from build123d import *

# Parameters (mm, degrees)
CROQUIS1_W              = 109.11
CROQUIS1_H              = 92
SALIENTE_EXTRUIR1_DEPTH = 32
CROQUIS2_W              = 86
CROQUIS2_H              = 27
CORTAR_EXTRUIR1_DEPTH   = 123.658029089
CORTAR_EXTRUIR2_DEPTH   = 107.753210842
CORTAR_EXTRUIR4_DEPTH   = 77.297103648


with BuildPart() as part:
    # Croquis1 → Saliente-Extruir1 (new body)
    with BuildSketch(Plane(origin=(0, 0, 0), x_dir=(1, 0, 0), z_dir=(0, 1, 0))):
        Rectangle(CROQUIS1_W, CROQUIS1_H)
    extrude(amount=SALIENTE_EXTRUIR1_DEPTH)

    # Croquis2 → Cortar-Extruir1 (cut, through all)
    with BuildSketch(Plane(origin=(54.555, 0, 0), x_dir=(0, 0, -1), z_dir=(1, 0, 0))):
        with Locations((-3, 18.5)):
            Rectangle(CROQUIS2_W, CROQUIS2_H)
    extrude(amount=-CORTAR_EXTRUIR1_DEPTH, mode=Mode.SUBTRACT)

    # Croquis3 → Cortar-Extruir2 (cut, through all)
    with BuildSketch(Plane.XY.offset(-40)):
        with BuildLine():
            Line((45.735, 28.9), (54.555, 28.9))
            Line((54.555, 28.9), (54.555, 25.1))
            Line((54.555, 25.1), (45.735, 25.1))
            ThreePointArc((45.735, 25.1), (43.835, 27), (45.735, 28.9))
        make_face()
        with BuildLine():
            Line((-45.735, 28.9), (-54.555, 28.9))
            Line((-54.555, 28.9), (-54.555, 25.1))
            Line((-54.555, 25.1), (-45.735, 25.1))
            ThreePointArc((-45.735, 25.1), (-43.835, 27), (-45.735, 28.9))
        make_face()
    extrude(amount=-CORTAR_EXTRUIR2_DEPTH, mode=Mode.SUBTRACT)

    # Croquis4 → Cortar-Extruir4 (cut, through all)
    with BuildSketch(Plane(origin=(0, 5, 0), x_dir=(1, 0, 0), z_dir=(0, 1, 0))):
        with BuildLine():
            Line((-46.015, 36), (-54.555, 36))
            Line((-54.555, 36), (-54.555, 31.26))
            Line((-54.555, 31.26), (-46.015, 31.26))
            ThreePointArc((-46.015, 31.26), (-43.645, 33.63), (-46.015, 36))
        make_face()
        with BuildLine():
            Line((-46.015, 17), (-54.555, 17))
            Line((-54.555, 17), (-54.555, 12.26))
            Line((-54.555, 12.26), (-46.015, 12.26))
            ThreePointArc((-46.015, 12.26), (-43.645, 14.63), (-46.015, 17))
        make_face()
        with BuildLine():
            Line((-46.015, -33.037861791), (-54.555, -33.037861791))
            Line((-54.555, -33.037861791), (-54.555, -37.615607647))
            Line((-54.555, -37.615607647), (-46.015, -37.615607647))
            ThreePointArc((-46.015, -37.615607647), (-43.726127072, -35.326734719), (-46.015, -33.037861791))
        make_face()
        with BuildLine():
            Line((54.555, -37.615607647), (46.015, -37.615607647))
            ThreePointArc((46.015, -37.615607647), (43.726127072, -35.326734719), (46.015, -33.037861791))
            Line((46.015, -33.037861791), (54.555, -33.037861791))
            Line((54.555, -33.037861791), (54.555, -37.615607647))
        make_face()
        with BuildLine():
            Line((54.555, 17), (54.555, 12.26))
            Line((54.555, 12.26), (46.015, 12.26))
            ThreePointArc((46.015, 12.26), (43.645, 14.63), (46.015, 17))
            Line((46.015, 17), (54.555, 17))
        make_face()
        with BuildLine():
            Line((54.555, 31.26), (46.015, 31.26))
            ThreePointArc((46.015, 31.26), (43.645, 33.63), (46.015, 36))
            Line((46.015, 36), (54.555, 36))
            Line((54.555, 36), (54.555, 31.26))
        make_face()
    extrude(amount=-CORTAR_EXTRUIR4_DEPTH, mode=Mode.SUBTRACT)


solid = part.part
Read the model definition and answer for the solid it produces. Units are mm, in the model's axes. A direction names the side the tool comes from. Give positions to 0.01 mm unless a question says otherwise; leave off trailing zeros. Write each loop counter-clockwise with the first axis right and the second up, starting at its lowest first coordinate (ties: lowest second). Pieces come first, ordered by that corner, then holes. Notation, with made-up numbers: (8.5, 56) -> (16.5, 56) arc R11 cw to (16.5, 62) -> close; hole circle Ø10 at (-4.5, 71). An arc over 180 degrees is marked (long way). Answer as a JSON object with one key per item and string values. Group by question number.
1) Find section B-B (z = 13.5). Write down the section's boundary in (x, y) (3 decimals).
2) Find section A-A (y = 3). Write down the section's boundary in (x, z) (3 decimals), and give its area (3 significant figures).
3) Consider L1, parallel to Y at x = -36.5, z = 28.5; L2, parallel to Z at x = -16.5, y = 19.5. Determine where each line is inside the solid, lowest interval first. Write a range as from..to.
4) Find section C-C (y = 27). Write down the section's boundary in (x, z) (3 decimals), and give its area (3 significant figures).
5) The mould has two halves that part along Y. Classify faces 4 (the flat face through (1, 5, 4)), 5 (the flat face through (-50, 25.1, -43)), 6 (the flat face through (54.555, 10, -42)): +Y half, -Y half, draft (parallel to the pull), parting line (faces both ways), or undercut.
6) A tool of negligible diameter and unlimited length cuts with its end or side. For faces 1 (the flat face through (1, 18, -40)), 2 (the flat face through (-50, 3, 33.038)), 3 (the flat face through (50, 3, -12.26)), from which of +Z, -Z, +X, -X, +Y, -Y can it reach the whole face along a straight path? Write none if from no direction.
7) Each of these flat-tipped pins is pushed along its axis until it touches: P1, Ø12, axis at x = -1.5, z = 36, coming from the +Y side; P2, Ø6, axis at x = -40.5, y = 9, coming from the +Z side; P3, Ø12, axis at y = 12.5, z = 1.5, coming from the -X side. Where does it stop, or does it pass through?
Values follow:
{
 "1": {"outline": "(-54.555, 0) -> (54.555, 0) -> (54.555, 5) -> (-54.555, 5) -> close"},
 "2": {"outline": "(-54.555, -46) -> (54.555, -46) -> (54.555, -36) -> (46.015, -36) arc R2.37 cw to (46.015, -31.26) -> (54.555, -31.26) -> (54.555, -17) -> (46.015, -17) arc R2.37 cw to (46.015, -12.26) -> (54.555, -12.26) -> (54.555, 33.038) -> (46.015, 33.038) arc R2.289 cw to (46.015, 37.616) -> (54.555, 37.616) -> (54.555, 46) -> (-54.555, 46) -> (-54.555, 37.616) -> (-46.015, 37.616) arc R2.289 cw to (-46.015, 33.038) -> (-54.555, 33.038) -> (-54.555, -12.26) -> (-46.015, -12.26) arc R2.37 cw to (-46.015, -17) -> (-54.555, -17) -> (-54.555, -31.26) -> (-46.015, -31.26) arc R2.37 cw to (-46.015, -36) -> (-54.555, -36) -> close", "area": "9,750 mm2"},
 "3": {"L1": "y = 0..5", "L2": "z = -46..-40"},
 "4": {"outline": "(-43.835, -46) -> (43.835, -46) -> (43.835, -40) -> (-43.835, -40) -> close", "area": "526 mm2"},
 "5": {"face 4": "+Y half", "face 5": "undercut", "face 6": "draft"},
 "6": {"face 1": "+Z, +X, -X, +Y", "face 2": "-X, +Y, -Y", "face 3": "+X, +Y, -Y"},
 "7": {"P1": "stops at y = 5", "P2": "stops at z = -40", "P3": "passes through"}
}
